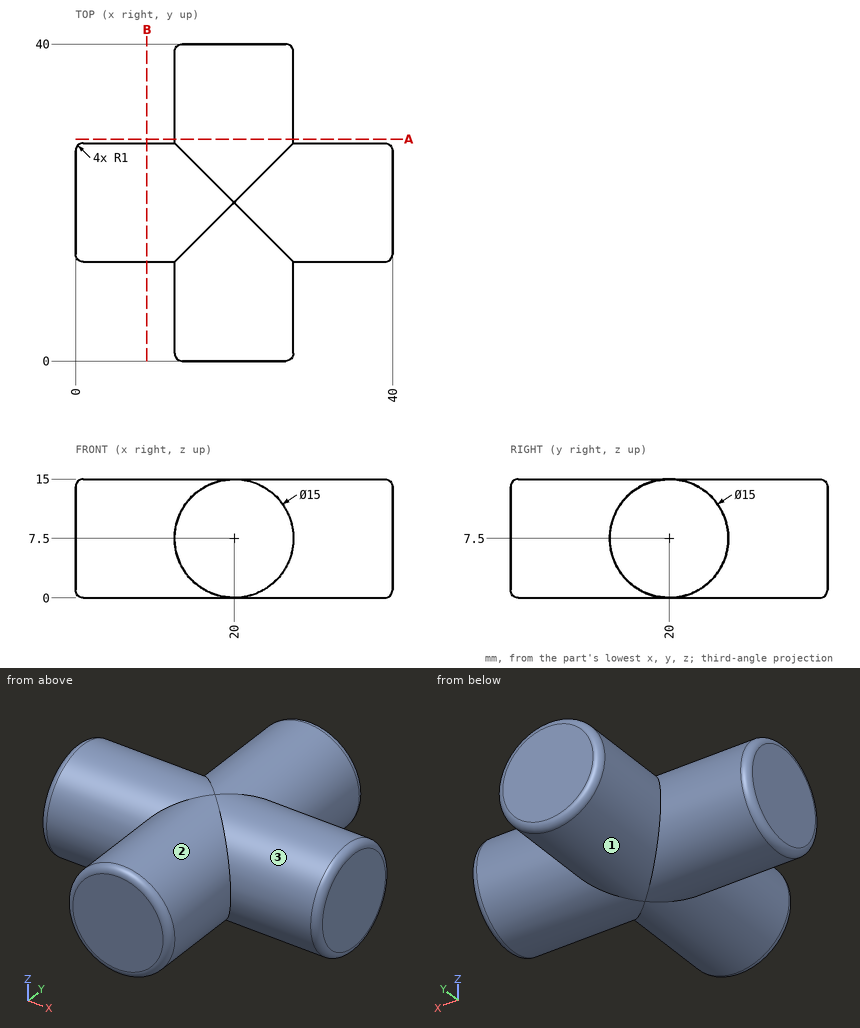
Can you work these out from the drawing? Everything is in mm from the part's minimum corner. A direction names the side the tool comes from. Round coordinates to 2 decimals unless told otherwise and drop trailing zeros. Loops run counter-clockwise (first coordinate to the right, second up) from the corner with the lowest first, then second, coordinate; pieces in that order, holes last. Notation, with made-up numbers: M 45,-38.75 L 99,-38.75 A23 ccw 99,-28.75 Z; hole C 76.25,89 d5. An arc over 180 degrees is marked long. Write item = value, one per line.
1. I need wall thicknesses on probe 1 along Y at (x, z) = (6.5, 7.5); probe 2 along Y at (x, z) = (2, 10.5); probe 3 along Z at (x, y) = (27, 26). Which ranges of each line are inside material? Lowest first, please.
Results below:
probe_1 = 12.5 to 27.5
probe_2 = 13.13 to 26.87
probe_3 = 3 to 12
2. Will these pins go through, and if not, where does the flat tip stop? P1, Ø1.5, axis at x = 13, z = 10, coming from the +Y side; P2, Ø8, axis at x = 10.5, y = 13, coming from the +Z side; P3, Ø1, axis at y = 4.5, z = 6, coming from the -X side.
Results below:
P1 = 39.98
P2 = 14.37
P3 = 12.57
3. Which directions (+Z, -Z, +X, -X, +Y, -Y) give clear straight access to the entire face, cutting with the end or side of a thin tool? Please do the marked faces 1, 2 and 3.
Results below:
face_1 = +Y
face_2 = -Y
face_3 = +X
4. I want a section at A-A, the plane y = 28. Write out the boundary of the cut face in (x, z).
Results below:
outline = C 20,7.5 d15
